Verification items for the finished model (mm, model axes). Face numbers are marked on the shaded views. A direction names the side the tool comes from. Give positions to 0.01 mm unless a question says otherwise; leave off trailing zeros. Write each loop counter-clockwise with the first axis right and the second up, starting at its lowest first coordinate (ties: lowest second). Pieces come first, ordered by that corner, then holes. Notation, with made-up numbers: (64, 31) -> (116, 31) arc R10 cw to (116, 38) -> close; hole circle Ø9 at (87.5, 51). An arc over 180 degrees is marked (long way). Write item = value, one per line.
Autodesk Inventor part; units mm, degrees
ref_plane "YZ Plane" through (0, 0, 0) normal (1, 0, 0) x (0, 1, 0)
ref_plane "XZ Plane" through (0, 0, 0) normal (0, 1, 0) x (-1, 0, 0)
ref_plane "XY Plane" through (0, 0, 0) normal (0, 0, 1) x (1, 0, 0)
sketch "Sketch1" plane through (0, 0, 0) normal (0, 1, 0) x (-1, 0, 0)
  line L0 (20, 14.965) -> (-20, 14.965)
  line L1 (-20, 14.965) -> (-20, -14.965)
  line L2 (-20, -14.965) -> (20, -14.965)
  line L3 (20, -14.965) -> (20, 14.965)
  point P0 (0, 0)
  dimension "d0" = 29.93
  dimension "d1" = 40
  dimension "d2" = 20
  dimension "d3" = 14.965
extrude "Plate1" add sketch "Sketch1" along normal blind 1.5
sketch "Sketch2" plane through (-20, 0, -13.465) normal (0, 0, -1) x (-1, 0, 0)
  line L0 (-40, 0) -> (0, 0)
  line L1 (0, 0) -> (0, 43.5)
  line L2 (0, 43.5) -> (-40, 43.5)
  line L3 (-40, 43.5) -> (-40, 0)
edge flange "Flange1" height 43.5 angle 90 thickness 1.5 bend radius 0.31 thickness toward (0, 0, -1) relief tear relief width 1.5 relief depth 0.75 corner gap 0.31 corner form 0 edges at (0, 1.5, -14.965) (0, 1.5, 14.965) wall of the first edge with corners at (20, 0, -13.465) (-20, 0, -13.465) (-20, 43.5, -13.465) (20, 43.5, -13.465)
bend "Bend1"
corner "Corner1"
sketch "Sketch3" plane through (-20, 43.5, 14.965) normal (0, 0, 1) x (1, 0, 0)
  line L0 (0, 0) -> (40, 0)
  line L1 (0, -41.69) -> (0, 0)
  circle A0 centre (20, -10) radius 10
  line L2 (0, -28.19) -> (40, -28.19)
  line L3 (40, -28.19) -> (40, -38.19)
  line L4 (40, -38.19) -> (0, -38.19)
  line L5 (0, -38.19) -> (0, -28.19)
  line L6 (40, -28.19) -> (28.9876, -5.6156)
  line L7 (0, -28.19) -> (11.0124, -5.6156)
  line L8 (0, 0) -> (40, 0)
  line L9 (40, 0) -> (40, -35)
  line L10 (40, -35) -> (0, -35)
  line L11 (0, -35) -> (0, 0)
  point P0 (20, -43.5)
  point P1 (20, 0)
  point P2 (0, -28.19)
  point P3 (0, -35)
  point P4 (30, -10)
  dimension "d15" = 10
  dimension "d16" = 0
  dimension "d17" = 20
  dimension "d18" = 18.19
  dimension "d19" = 0
  dimension "d20" = 40
  dimension "d21" = 10
  dimension "d22" = 35
extrude "Extrusion1" cut sketch "Sketch3" against normal blind 35 contours L0 A0 L7 L1 | L0 L9 L6 A0
sketch "Sketch4" plane through (20, 1.81, -14.965) normal (0, 0, -1) x (-1, 0, 0)
  arc A0 (28.9876, 36.0744) -> (11.0124, 36.0744) centre (20, 31.69) ccw
  circle A1 centre (20, 31.69) radius 2.6
  circle A2 centre (13, 31.69) radius 1.05
  circle A3 centre (27, 31.69) radius 1.05
  circle A4 centre (20, 38.69) radius 1.05
  circle A5 centre (20, 24.69) radius 1.05
  point P0 (20, -1.81)
  dimension "d25" = 5.2
  dimension "d26" = 0
  dimension "d27" = 7
  dimension "d28" = 2.1
  dimension "d29" = 7
  dimension "d30" = 0
  dimension "d31" = 2.1
  dimension "d32" = 0
  dimension "d33" = 7
  dimension "d34" = 2.1
  dimension "d35" = 7
  dimension "d36" = 0
  dimension "d37" = 2.1
extrude "Extrusion2" cut sketch "Sketch4" against normal blind 1.5
sketch "Sketch5" plane through (-20, 1.81, 14.965) normal (0, 0, 1) x (1, 0, 0)
  arc A0 (28.9876, 36.0744) -> (11.0124, 36.0744) centre (20, 31.69) ccw
  circle A1 centre (20, 31.69) radius 2.55
  point P0 (20, -1.81)
  dimension "d40" = 5.1
extrude "Extrusion3" cut sketch "Sketch5" against normal blind 1.5
sketch "Sketch6" plane through (0, 1.5, 0) normal (0, 1, 0) x (1, 0, 0)
  circle A0 centre (-14, -10.155) radius 1.05
  circle A1 centre (-14, -0.75) radius 1.05
  circle A2 centre (-14, 8.655) radius 1.05
  circle A3 centre (14, -10.155) radius 1.05
  circle A4 centre (14, -0.75) radius 1.05
  circle A5 centre (14, 8.655) radius 1.05
  point P0 (0, 0)
hole "Hole1" at (14, 1.5, -8.655) at (14, 1.5, 0.75) at (14, 1.5, 10.155) at (-14, 1.5, 10.155) at (-14, 1.5, 0.75) at (-14, 1.5, -8.655) direction (0, -1, 0) diameter 2.1 depth 1.5
equation "\"d48\" = Thickness"
equation "\"d4\" = Thickness"
equation "\"d5\" = BendReliefWidth"
equation "\"d6\" = BendReliefDepth"
equation "\"d7\" = MinimumRemnant"
equation "\"d8\" = TransitionRadius"
equation "\"d11\" = BendRadius"
equation "\"d12\" = CornerReliefSize"
equation "\"d13\" = GapSize"
equation "\"d14\" = JacobiRadiusSize"
equation "\"BendReliefWidth\" = Thickness"
equation "\"BendReliefDepth\" = 0.5 * Thickness"
equation "\"CornerReliefSize\" = 4 * Thickness"
equation "\"MinimumRemnant\" = 2 * Thickness"
equation "\"TransitionRadius\" = BendRadius"
equation "\"JacobiRadiusSize\" = BendRadius"
equation "\"GapSize\" = Thickness"
properties part number "partpart" material "Aluminum 6061-AHC"
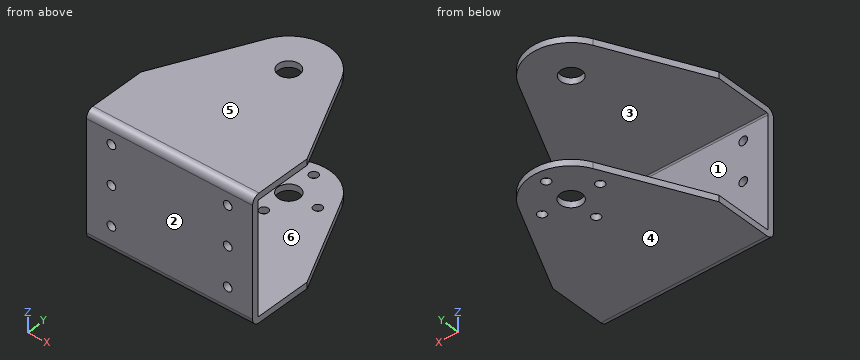
Item 1: Mould release check, pull along Z, two halves, no side actions. Record for the marked faces 1, 2, 3 and 4: +Z half, -Z half, draft (parallel to the pull), parting line (faces both ways), or undercut.
Response values:
face_1 = undercut
face_2 = draft
face_3 = undercut
face_4 = -Z half
Item 2: Material ranges on line 1 (Z direction, x = 10, y = 27) (3 decimals); line 2 (Z direction, x = -14, y = 0.9) (3 decimals); line 3 (Y direction, x = 6.5, z = -9.5), recorded low to high.
Response values:
line_1 = -14.965 to -13.465, 13.465 to 14.965
line_2 = -14.72 to -9.705, -7.605 to -0.3, 1.8 to 9.105, 11.205 to 14.72
line_3 = 0 to 1.5
Item 3: Sectioned sample at D-D on x = 14. Record the cut outline in (y, z) (3 decimals), then the cut area to 3 significant figures.
Response values:
outline = (0, -13.155) arc R1.81 ccw to (1.81, -14.965) -> (27.609, -14.965) -> (27.609, -13.465) -> (1.81, -13.465) arc R0.31 cw to (1.5, -13.155) -> (1.5, -9.705) -> (0, -9.705) -> close; (0, -7.605) -> (1.5, -7.605) -> (1.5, -0.3) -> (0, -0.3) -> close; (0, 1.8) -> (1.5, 1.8) -> (1.5, 9.105) -> (0, 9.105) -> close; (0, 11.205) -> (1.5, 11.205) -> (1.5, 13.155) arc R0.31 cw to (1.81, 13.465) -> (27.609, 13.465) -> (27.609, 14.965) -> (1.81, 14.965) arc R1.81 ccw to (0, 13.155) -> close
area = 112 mm^2
Item 4: Sectioned sample at C-C on y = 26.5. Record the cut outline in (x, z) (3 decimals).
Response values:
outline = (-14.541, -14.965) -> (-1.05, -14.965) -> (-1.05, -13.465) -> (-14.541, -13.465) -> close; (-14.541, 13.465) -> (14.541, 13.465) -> (14.541, 14.965) -> (-14.541, 14.965) -> close; (1.05, -14.965) -> (14.541, -14.965) -> (14.541, -13.465) -> (1.05, -13.465) -> close
Item 5: Go/stop test with flat-tipped pins: P1, Ø2.5, axis at x = 7, y = 33.5, coming from the -Z side (3 decimals); P2, Ø2.5, axis at x = -14, z = 10.155, coming from the +Y side; P3, Ø1.3, axis at x = -7, y = 33.5, coming from the -Z side (3 decimals). Record where each tip stops, or that it passes through.
Response values:
P1 = -14.965
P2 = 1.5
P3 = 13.465
Item 6: Set-up check for the marked faces 5 and 6: record each of +Z, -Z, +X, -X, +Y, -Y from which the full face is reachable in a straight line by a thin tool's end or side.
Response values:
face_5 = +Z, +X, -X, +Y, -Y
face_6 = +X, -X, +Y
Item 7: Sectioned sample at B-B on x = 7. Record the cut outline in (y, z) (3 decimals).
Response values:
outline = (0, -13.155) arc R1.81 ccw to (1.81, -14.965) -> (32.45, -14.965) -> (32.45, -13.465) -> (1.81, -13.465) arc R0.31 cw to (1.5, -13.155) -> (1.5, 13.155) arc R0.31 cw to (1.81, 13.465) -> (40.641, 13.465) -> (40.641, 14.965) -> (1.81, 14.965) arc R1.81 ccw to (0, 13.155) -> close; (34.55, -14.965) -> (40.641, -14.965) -> (40.641, -13.465) -> (34.55, -13.465) -> close
Item 8: Sectioned sample at A-A on z = 0.75. Record the cut outline in (x, y), then the cut area to 3 significant figures.
Response values:
outline = (-20, 0) -> (-15.05, 0) -> (-15.05, 1.5) -> (-20, 1.5) -> close; (-12.95, 0) -> (12.95, 0) -> (12.95, 1.5) -> (-12.95, 1.5) -> close; (15.05, 0) -> (20, 0) -> (20, 1.5) -> (15.05, 1.5) -> close
area = 53.7 mm^2
